Autodesk Inventor part; units mm, degrees
ref_plane "YZ Plane" through (0, 0, 0) normal (1, 0, 0) x (0, 1, 0)
ref_plane "XZ Plane" through (0, 0, 0) normal (0, 1, 0) x (-1, 0, 0)
ref_plane "XY Plane" through (0, 0, 0) normal (0, 0, 1) x (1, 0, 0)
sketch "Sketch1" plane through (0, 0, 0) normal (0, 1, 0) x (-1, 0, 0)
  circle A0 centre (0, 0) radius 14.5 construction
  circle A1 centre (0, 0) radius 2.5
  line L0 (-4, 0.5) -> (-1, 0.5)
  line L1 (-1, 0.5) -> (-1, -0.5)
  line L2 (-1, -0.5) -> (-4, -0.5)
  line L3 (-4, -0.5) -> (-4, 0.5)
  line L4 (-4, 0.5) -> (-1, -0.5) construction
  line L5 (-1, 0.5) -> (-4, -0.5) construction
  line L6 (20, 20) -> (-20, 20)
  line L7 (-20, 20) -> (-20, -20)
  line L8 (-20, -20) -> (20, -20)
  line L9 (20, -20) -> (20, 20)
  line L10 (20, 20) -> (-20, -20) construction
  line L11 (-20, 20) -> (20, -20) construction
  point P0 (-2.5, 0)
  point P1 (-2.4495, 0.5)
  point P2 (-2.4495, -0.5)
  dimension "d1" = 5
  dimension "d0" = 29
  dimension "d2" = 1
  dimension "d3" = 1
  dimension "d6" = 40
  dimension "d7" = 40
extrude "Extrusion1" add sketch "Sketch1" along normal blind 3 contours L0 L1 L2 A1 | A1 L2 L3 L0 | L9 L8 L7 L6 picked at (-1.4981, -0.0559)
sketch "Sketch2" plane through (0, 3, 0) normal (0, 1, 0) x (1, 0, 0)
  arc A0 (2.4495, 0.5) -> (2.4495, -0.5) centre (0, 0) ccw
  line L0 (-20, 20) -> (-20, -20)
  circle A1 centre (0, 0) radius 20 construction
  line L1 (-20, -20) -> (0, 0) construction
  point P0 (-14.1421, -14.1421)
  point P1 (14.1421, -14.1421)
  point P2 (14.1421, 14.1421)
  point P3 (-14.1421, 14.1421)
  dimension "d8" = 40
  dimension "d11" = 360
hole "Hole1" at (-14.1421, 3, 14.1421) at (14.1421, 3, 14.1421) at (14.1421, 3, -14.1421) at (-14.1421, 3, -14.1421) direction (0, -1, 0) diameter 3.4 end through all
fillet "Fillet1" radius 5 4 edges at (-20, 1.5, 20) (-20, 1.5, -20) (20, 1.5, -20) (20, 1.5, 20)
equation "\"d7\" = d6"
properties part number "rod allingment"
Input: part model. Units: mm. Frame: model coordinates. A direction names the side the tool comes from. Give positions to 0.01 mm unless a question says otherwise; leave off trailing zeros. Order: outer loops, then holes, each group sorted by start corner. A loop starts at its lowest first (then second) coordinate and runs counter-clockwise, first axis right, second up. Notation, with made-up numbers: M 67.5,14 L 118.5,14 A21 cw 118.5,23 Z; hole C -16.75,52.5 d6. An arc over 180 degrees is marked long. Answer as a JSON object with one key per item and string values.
1. Ray query, line 1 (X direction, y = 2.1, z = 14); line 2 (X direction, y = 1.1, z = 0); line 3 (X direction, y = 1.5, z = 15). Return the intervals inside material, ascending. Write a range as [from, to].
Result sheet:
{"line 1": "[-20, -15.84], [-12.45, 12.45], [15.84, 20]", "line 2": "[-20, -2.5], [1, 20]", "line 3": "[-20, -15.61], [-12.67, 12.67], [15.61, 20]"}
2. Cut plane C-C, the plane x = -13. Output: boundary loops of the cut face in (y, z), and give its area (3 significant figures).
Result sheet:
{"outline": "M 0,-20 L 3,-20 L 3,-15.4 L 0,-15.4 Z; M 0,-12.88 L 3,-12.88 L 3,12.88 L 0,12.88 Z; M 0,15.4 L 3,15.4 L 3,20 L 0,20 Z", "area": "105 mm²"}
3. First-contact query: P1, Ø2.5, axis at x = -14.14, z = -14.14, coming from the -Y side. Flat tip, straight axial feed; report the tip coordinate or a pass-through.
Result sheet:
{"P1": "through"}
4. Reachability of faces 4 (the cylindrical face through (19, 2, -18)), 5 (the flat face through (2, 1, -0.5)) from +Z, -Z, +X, -X, +Y, -Y: full face, straight path, thin tool, end or side. Return the list, or none.
Result sheet:
{"face 4": "-Z, +X, +Y, -Y", "face 5": "+Y, -Y"}
5. Cut plane D-D, the plane y = 2.45. Output: boundary loops of the cut face in (x, z), and give its area (3 significant figures).
Result sheet:
{"outline": "M -20,-15 A5 ccw -15,-20 L 15,-20 A5 ccw 20,-15 L 20,15 A5 ccw 15,20 L -15,20 A5 ccw -20,15 Z; hole C -14.14,-14.14 d3.4; hole C -14.14,14.14 d3.4; hole M 1,-0.5 L 1,0.5 L 2.45,0.5 A2.5 ccw long 2.45,-0.5 Z; hole C 14.14,-14.14 d3.4; hole C 14.14,14.14 d3.4", "area": "1,520 mm²"}
6. Cut plane A-A, the plane x = 0. Output: boundary loops of the cut face in (y, z), and give its area (3 significant figures).
Result sheet:
{"outline": "M 0,-20 L 3,-20 L 3,-2.5 L 0,-2.5 Z; M 0,2.5 L 3,2.5 L 3,20 L 0,20 Z", "area": "105 mm²"}
7. Cut plane B-B, the plane z = 0. Output: boundary loops of the cut face in (x, y), and give its area (4 significant figures).
Result sheet:
{"outline": "M -20,0 L -2.5,0 L -2.5,3 L -20,3 Z; M 1,0 L 20,0 L 20,3 L 1,3 Z", "area": "109.5 mm²"}
8. Pull-direction query (X, two-part tool) for faces 1 (the flat face through (-4, 3, 0)), 2 (the cylindrical face through (-19, 2, 18)), 3 (the cylindrical face through (-13.108, 1.479, -15.491)); classes: +X half, -X half, draft (parallel to the pull), parting line (faces both ways), or undercut.
Result sheet:
{"face 1": "draft", "face 2": "-X half", "face 3": "undercut"}
